Can you work these out from the model? Positions are in its coordinate system, mm. Round coordinates to 2 decimals unless told otherwise and drop trailing zeros. Order: outer loops, then holes, each group sorted by start corner. A loop starts at its lowest first (then second) coordinate and runs counter-clockwise, first axis right, second up. Notation, with made-up numbers: (65.25, 72.25) -> (119.25, 72.25) arc R20 cw to (119.25, 91.25) -> close; hole circle Ø3 at (33.25, 61). An arc over 180 degrees is marked (long way). One line per item, written item: value.
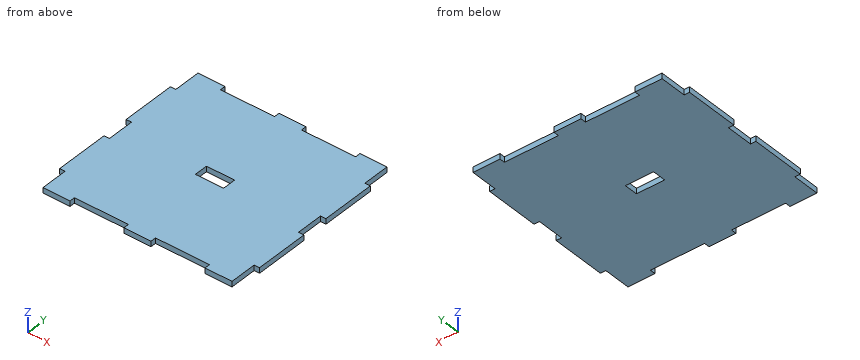
```python
from build123d import *

# Parameters (mm, degrees)
SKETCH1_W           = 70
SKETCH1_H           = 70
BOSS_EXTRUDE1_DEPTH = 2
SKETCH2_W           = 2
SKETCH2_H           = 20
BOSS_EXTRUDE2_DEPTH = 2
SKETCH3_W           = 20
SKETCH3_H           = 2
CUT_EXTRUDE1_DEPTH  = 2
SKETCH4_W           = 10.41
SKETCH4_H           = 5
CUT_EXTRUDE2_DEPTH  = 10


with BuildPart() as part:
    # Sketch1 → Boss-Extrude1 (new body)
    with BuildSketch(Plane.XY):
        Rectangle(SKETCH1_W, SKETCH1_H)
    extrude(amount=-BOSS_EXTRUDE1_DEPTH)

    # Sketch2 → Boss-Extrude2 (add)
    with BuildSketch(Plane.XY):
        with Locations((-36, 15)):
            Rectangle(SKETCH2_W, SKETCH2_H)
        with Locations((-36, -15)):
            Rectangle(SKETCH2_W, SKETCH2_H)
        with Locations((36, -15)):
            Rectangle(SKETCH2_W, SKETCH2_H)
        with Locations((36, 15)):
            Rectangle(SKETCH2_W, SKETCH2_H)
    extrude(amount=-BOSS_EXTRUDE2_DEPTH)

    # Sketch3 → Cut-Extrude1 (cut)
    with BuildSketch(Plane.XY):
        with Locations((-15, 34)):
            Rectangle(SKETCH3_W, SKETCH3_H)
        with Locations((15, 34)):
            Rectangle(SKETCH3_W, SKETCH3_H)
        with Locations((-15, -34)):
            Rectangle(SKETCH3_W, SKETCH3_H)
        with Locations((15, -34)):
            Rectangle(SKETCH3_W, SKETCH3_H)
    extrude(amount=-CUT_EXTRUDE1_DEPTH, mode=Mode.SUBTRACT)

    # Sketch4 → Cut-Extrude2 (cut)
    with BuildSketch(Plane.XY):
        Rectangle(SKETCH4_W, SKETCH4_H)
    extrude(amount=-CUT_EXTRUDE2_DEPTH, mode=Mode.SUBTRACT)


solid = part.part
```
Q1. Will these pins go through, and if not, where does the flat tip stop? pin 1 Ø1 at (y, z) = (0, -0.5) entering from +X; pin 2 Ø0.6 at (y, z) = (34.5, -1.5) entering from -X; pin 3 Ø0.6 at (x, z) = (-35.5, -1) entering from -Y.
Answers below:
pin 1: x = 35
pin 2: x = -35
pin 3: y = -25
Q2. Please list where these lines run through material, in increasing order: line 1 along Y through (x, z) = (4, -1.4); line 2 along Y through (x, z) = (10, -1.45); line 3 along X through (y, z) = (26, -1.8).
Answers below:
line 1: -35 to -2.5, 2.5 to 35
line 2: -33 to 33
line 3: -35 to 35
Q3. I want a section at C-C on x = -12.5. List the corners of the cut face in (y, z) for me.
Answers below:
outline: (-33, -2) -> (33, -2) -> (33, 0) -> (-33, 0) -> close
Q4. I want a section at A-A on x = 0. List the corners of the cut face in (y, z) for me, plus the area to 3 significant figures.
Answers below:
outline: (-35, -2) -> (-2.5, -2) -> (-2.5, 0) -> (-35, 0) -> close; (2.5, -2) -> (35, -2) -> (35, 0) -> (2.5, 0) -> close
area: 130 mm^2
Q5. I want a section at B-B on y = -1.5. List the corners of the cut face in (x, z) for me (3 decimals).
Answers below:
outline: (-35, -2) -> (-5.205, -2) -> (-5.205, 0) -> (-35, 0) -> close; (5.205, -2) -> (35, -2) -> (35, 0) -> (5.205, 0) -> close
